For this review, take the finished solid that the model builds, in its own axes (mm). Face numbers are marked on the shaded views. A direction names the side the tool comes from. Give positions to 0.01 mm unless a question says otherwise; leave off trailing zeros. Write each loop counter-clockwise with the first axis right and the second up, starting at its lowest first coordinate (ties: lowest second). Pieces come first, ordered by that corner, then holes.
1) We need section C-C on x = 19. Give the boundary of the cut face in (y, z).
2) Machinability: for the marked faces 1, 2, 3, 4 and 5, which of the approach directions +Z, -Z, +X, -X, +Y, -Y give a long, thin tool a straight path to every point of the face, cutting with its end or side? Answer none if there is none.
3) For P1, Ø1, axis at y = -3.5, z = -6, coming from the -X side, flat-tipped, find the tip position at first contact; note if it passes through.
4) We need section B-B on x = 23.5. Give the boundary of the cut face in (y, z), and give its area (3 significant figures).
5) We need section A-A on z = 1.5. Give the boundary of the cut face in (x, y), and give its area (3 significant figures).
6) Draft analysis for pull direction Z (two halves, no side actions). For the marked faces 6, 7, 8 and 9, state which applies: pulls with the +Z half, pulls with the -Z half, needs draft (parallel to the pull), parting line crosses it, or undercut.
from build123d import *

# Parameters (mm, degrees)
SKETCH1_W           = 12
SKETCH1_H           = 16
SKETCH1_R           = 2.1
SKETCH1_W_2         = 2
BOSS_EXTRUDE1_DEPTH = 22
FILLET1_R           = 5
SKETCH2_W           = 9
SKETCH2_H           = 1.9
BOSS_EXTRUDE2_DEPTH = 5
SKETCH4_W           = 12
SKETCH4_H           = 22
BOSS_EXTRUDE3_DEPTH = 9.13
FILLET2_R           = 5.1
SKETCH5_W           = 3
SKETCH5_H           = 8
BOSS_EXTRUDE4_DEPTH = 8
FILLET3_R           = 2
BOSS_EXTRUDE5_DEPTH = 10
BOSS_EXTRUDE6_DEPTH = 12.016468152
FILLET4_R           = 5
FILLET5_R           = 2
FILLET6_R           = 5


with BuildPart() as part:
    # Sketch1 → Boss-Extrude1 (new body)
    # profile 1 of 2: a face of its own
    with BuildSketch(Plane(origin=(0, 0, 0), x_dir=(1, 0, 0), z_dir=(0, 1, 0))):
        Rectangle(SKETCH1_W, SKETCH1_H)
        with Locations(Location((0, 0, 0), (0, 0, 270))):
            Circle(SKETCH1_R, mode=Mode.SUBTRACT)
    # profile 2 of 2: a face of its own
    with BuildSketch(Plane(origin=(0, 0, 0), x_dir=(1, 0, 0), z_dir=(0, 1, 0))):
        with Locations((7, 0)):
            Rectangle(SKETCH1_W_2, SKETCH1_H)
    extrude(amount=BOSS_EXTRUDE1_DEPTH)

    # Fillet1
    fillet1_edges = [part.edges().sort_by_distance(p)[0] for p in [
        (-6, 11, 8),
        (-6, 11, -8),
    ]]
    fillet(fillet1_edges, radius=FILLET1_R)

    # Sketch2 → Boss-Extrude2 (add)
    with BuildSketch(Plane(origin=(0, 22, 0), x_dir=(1, 0, 0), z_dir=(0, 1, 0))):
        with Locations((3.5, 7.05)):
            Rectangle(SKETCH2_W, SKETCH2_H)
        with Locations((3.5, -7.05)):
            Rectangle(SKETCH2_W, SKETCH2_H)
    extrude(amount=BOSS_EXTRUDE2_DEPTH)

    # Sketch4 → Boss-Extrude3 (add)
    with BuildSketch(Plane(origin=(8, 0, 0), x_dir=(0, 0, -1), z_dir=(1, 0, 0))):
        with Locations((0, 11)):
            Rectangle(SKETCH4_W, SKETCH4_H)
    extrude(amount=BOSS_EXTRUDE3_DEPTH)

    # Fillet2
    fillet2_edges = [part.edges().sort_by_distance(p)[0] for p in [
        (17.13, 22, 0),
    ]]
    fillet(fillet2_edges, radius=FILLET2_R)

    # Sketch5 → Boss-Extrude4 (add)
    with BuildSketch(Plane.XZ):
        with Locations((10.6, 0)):
            Rectangle(SKETCH5_W, SKETCH5_H)
    extrude(amount=BOSS_EXTRUDE4_DEPTH)

    # Fillet3
    fillet3_edges = [part.edges().sort_by_distance(p)[0] for p in [
        (10.6, 0, 4),
        (10.6, 0, -4),
    ]]
    fillet(fillet3_edges, radius=FILLET3_R - 0.0001)  # a hair under: the kernel refuses the full size

    # Sketch6 → Boss-Extrude5 (add)
    with BuildSketch(Plane(origin=(17.13, 0, 0), x_dir=(0, 0, -1), z_dir=(1, 0, 0))):
        Polygon((-6, 9.8), (6, 10.428893351), (6, 0), (-6, 0), align=None)
    extrude(amount=BOSS_EXTRUDE5_DEPTH)

    # Sketch8 → Boss-Extrude6 (add, along a direction that is not the sketch's normal)
    with BuildSketch(Plane.XY.offset(6)):
        Polygon((17.13, 9.8), (27.13, 10.324077793), (27.13, 9.8), align=None)
    extrude(amount=-BOSS_EXTRUDE6_DEPTH, dir=(0, -0.052335956242944494, 0.9986295347545739))

    # Fillet4
    fillet4_edges = [part.edges().sort_by_distance(p)[0] for p in [
        (12.1, 0, 0),
    ]]
    fillet(fillet4_edges, radius=FILLET4_R)

    # Fillet5
    fillet5_edges = [part.edges().sort_by_distance(p)[0] for p in [
        (-1, 22, -7.05),
        (-1, 22, 7.05),
        (8, 11, -6),
        (8, 11, 6),
    ]]
    fillet(fillet5_edges, radius=FILLET5_R - 0.0001)  # a hair under: the kernel refuses the full size

    # Fillet6
    fillet6_edges = [part.edges().sort_by_distance(p)[0] for p in [
        (27.13, 0, 0),
    ]]
    fillet(fillet6_edges, radius=FILLET6_R)


solid = part.part
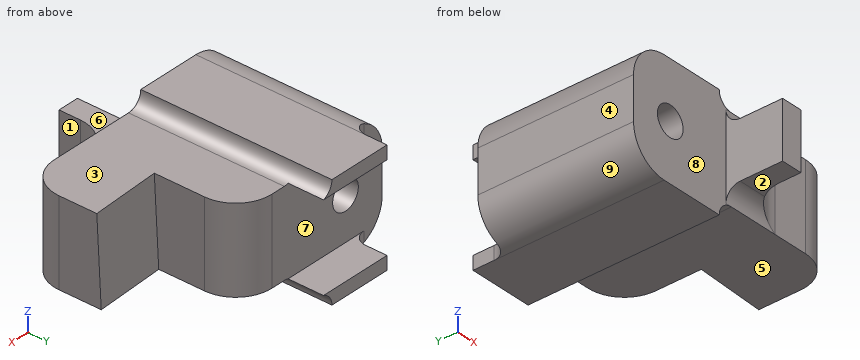
Results list:
1. outline: (0, -6) - (10.53, -6) - (9.9, 6) - (0, 6) - close
2. face 1: +Z, -Z, +X, -Y
2. face 2: -Z, +X, -X, -Y
2. face 3: +Z, +X, +Y, -Y
2. face 4: +Z, -Z, -X, +Y, -Y
2. face 5: -Z, +X, +Y, -Y
3. P1: passes through
4. outline: (0.19, -6) - (10.76, -6) - (10.13, 6) - (0.19, 6) - close
4. area: 123 mm2
5. outline: (-6, 0) - (-1.47, 0) - (-1.47, 22) - (-6, 22) - close; (1.47, 0) - (9.1, 0) - (9.1, -8) - (12.1, -8) - (12.1, -5) arc R5 cw to (17.1, 0) - (22.13, 0) arc R5 ccw to (27.13, 5) - (27.13, 10.56) - (17.13, 10.04) - (17.13, 16.9) arc R5.1 ccw to (12.03, 22) - (1.47, 22) - close
5. area: 566 mm2
6. face 6: pulls with the +Z half
6. face 7: undercut
6. face 8: needs draft
6. face 9: pulls with the -Z half
